```python
from build123d import *

# Parameters (mm, degrees)
SKETCH1_R           = 1.95
BOSS_EXTRUDE1_DEPTH = 60
SKETCH2_W           = 8
SKETCH2_H           = 3.9
BOSS_EXTRUDE2_DEPTH = 3.175
SKETCH3_R           = 0.75
CUT_EXTRUDE1_DEPTH  = 5


with BuildPart() as part:
    # Sketch1 → Boss-Extrude1 (new body)
    with BuildSketch(Plane.XY):
        Circle(SKETCH1_R)
    extrude(amount=BOSS_EXTRUDE1_DEPTH)

    # Sketch2 → Boss-Extrude2 (add)
    with BuildSketch(Plane.XY.offset(60)):
        Rectangle(SKETCH2_W, SKETCH2_H)
    extrude(amount=BOSS_EXTRUDE2_DEPTH)

    # Sketch3 → Cut-Extrude1 (cut)
    with BuildSketch(Plane(origin=(0, 1.95, 0), x_dir=(1, 0, 0), z_dir=(0, 1, 0))):
        with Locations((0, -7)):
            Circle(SKETCH3_R)
    extrude(amount=-CUT_EXTRUDE1_DEPTH, mode=Mode.SUBTRACT)


solid = part.part
```
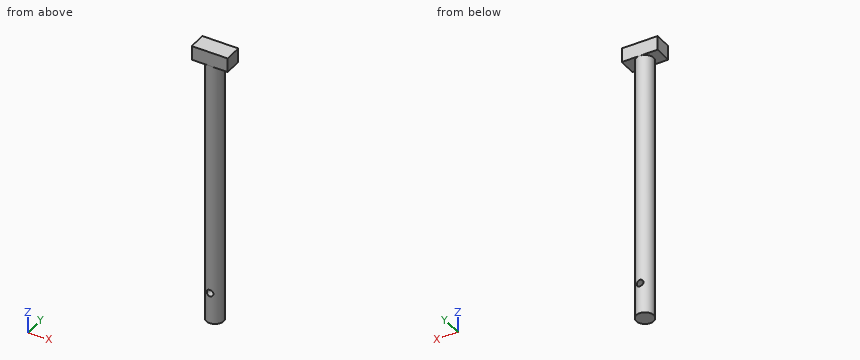
Could you check a few things on this model? Use its own coordinates, in mm. Round coordinates to 2 decimals unless told otherwise and drop trailing zeros. Loops run counter-clockwise (first coordinate to the right, second up) from the corner with the lowest first, then second, coordinate; pieces in that order, holes last. Notation, with made-up numbers: M 84,-0.5 L 95,-0.5 A26 cw 95,34.5 Z; hole C 13.5,51 d1. An arc over 180 degrees is marked long. Write item = value, one per line.
1. I need wall thicknesses on probe 1 along Z at (x, y) = (0, 1.05) (3 decimals); probe 2 along X at (y, z) = (-1.1, 7); probe 3 along X at (y, z) = (-0.2, 32.5). Which ranges of each line are inside material? Lowest first, please.
Results below:
probe_1 = 0 to 6.25, 7.75 to 63.175
probe_2 = -1.61 to -0.75, 0.75 to 1.61
probe_3 = -1.94 to 1.94
2. I want a section at A-A, the plane y = 0. Write out the boundary of the cut face in (x, z) (3 decimals).
Results below:
outline = M -4,60 L -1.95,60 L -1.95,0 L 1.95,0 L 1.95,60 L 4,60 L 4,63.175 L -4,63.175 Z; hole C 0,7 d1.5
3. Will these pins go through, and if not, where does the flat tip stop? P1, Ø1, axis at y = -0.5, z = 45.5, coming from the +X side; P2, Ø2, axis at x = 2, z = 21.5, coming from the -Y side; P3, Ø2, axis at x = -3, y = 0, coming from the -Z side.
Results below:
P1 = 1.95
P2 = -1.67
P3 = 60
4. I want a section at B-B, the plane z = 7. Write out the boundary of the cut face in (x, y).
Results below:
outline = M -0.75,-1.8 L -0.75,1.8 A1.95 ccw Z; M 0.75,-1.8 A1.95 ccw 0.75,1.8 Z
